Verification items for this drawing (mm, ordinates from the low corner). Coordinates: 2 decimals unless noted, no trailing zeros. Order: outer loops, then holes, each group sorted by start corner. A loop starts at its lowest first (then second) coordinate and runs counter-clockwise, first axis right, second up. Notation, with made-up numbers: (25, 32.5) -> (29, 32.5) arc R17 ccw to (29, 52.5) -> close; hole circle Ø1 at (45.5, 76.25). An arc over 180 degrees is marked (long way). Write item = value, one per line. Start each with the question number.
1. Cross-section at C-C on z = 9. Record the cut outline in (x, y), plus the area to 3 significant figures.
2. Go/stop test with flat-tipped pins: P1, Ø6, axis at x = 112.5, y = 5, coming from the -Z side; P2, Ø3, axis at x = 49.5, z = 8, coming from the +Y side. Record where each tip stops, or that it passes through.
3. Thickness scan on line 1 along X through (y, z) = (9, 13.65); line 2 along X through (y, z) = (1.25, 9); line 3 along Z through (x, y) = (132.5, 12.25). Record the ranges inside material, lowest first. Write a range as from..to.
4. Cross-section at D-D on x = 20. Record the cut outline in (y, z), plus the area to 3 significant figures.
5. Cross-section at B-B on x = 150. Record the cut outline in (y, z), plus the area to 3 significant figures.
6. Cross-section at A-A on y = 5.75. Record the cut outline in (x, z).
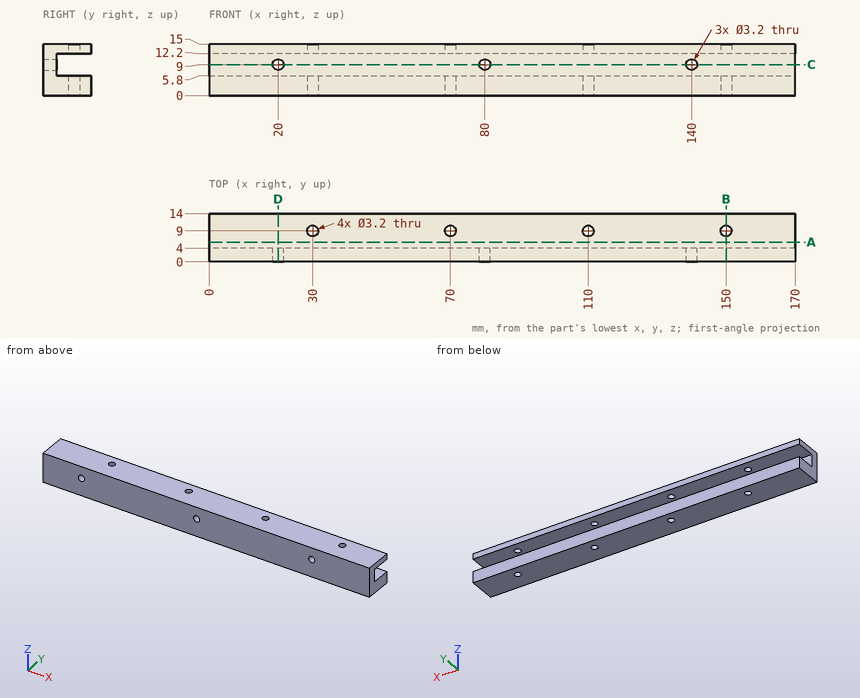
Worked out:
q1.outline = (0, 0) -> (18.4, 0) -> (18.4, 4) -> (0, 4) -> close; (21.6, 0) -> (78.4, 0) -> (78.4, 4) -> (21.6, 4) -> close; (81.6, 0) -> (138.4, 0) -> (138.4, 4) -> (81.6, 4) -> close; (141.6, 0) -> (170, 0) -> (170, 4) -> (141.6, 4) -> close
q1.area = 642 mm²
q2.P1 = 0
q2.P2 = 4
q3.line_1 = 0..28.4, 31.6..68.4, 71.6..108.4, 111.6..148.4, 151.6..170
q3.line_2 = 0..18.4, 21.6..78.4, 81.6..138.4, 141.6..170
q3.line_3 = 0..5.8, 12.2..15
q4.outline = (0, 0) -> (14, 0) -> (14, 5.8) -> (4, 5.8) -> (4, 7.4) -> (0, 7.4) -> close; (0, 10.6) -> (4, 10.6) -> (4, 12.2) -> (14, 12.2) -> (14, 15) -> (0, 15) -> close
q4.area = 133 mm²
q5.outline = (0, 0) -> (7.4, 0) -> (7.4, 5.8) -> (4, 5.8) -> (4, 12.2) -> (7.4, 12.2) -> (7.4, 15) -> (0, 15) -> close; (10.6, 0) -> (14, 0) -> (14, 5.8) -> (10.6, 5.8) -> close; (10.6, 12.2) -> (14, 12.2) -> (14, 15) -> (10.6, 15) -> close
q5.area = 118 mm²
q6.outline = (0, 0) -> (170, 0) -> (170, 5.8) -> (0, 5.8) -> close; (0, 12.2) -> (170, 12.2) -> (170, 15) -> (0, 15) -> close
